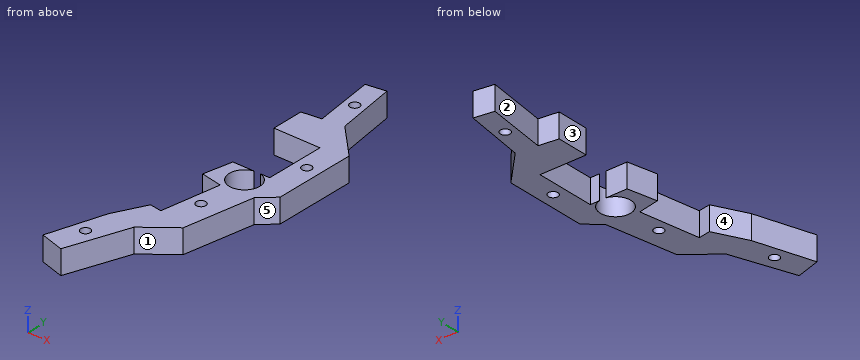
```python
from build123d import *

# Parameters (mm, degrees)
SKETCH1_R           = 1
BOSS_EXTRUDE1_DEPTH = 5
SKETCH2_R           = 3.2
CUT_EXTRUDE1_DEPTH  = 6


with BuildPart() as part:
    # Sketch1 → Boss-Extrude1 (new body)
    with BuildSketch(Plane.XY):
        Polygon((-30.344978495, 29.354997846), (-26.26481101, 29.998979434), (-24.229853855, 17.105806435), (-17.589395727, 10.355662433), (-17.589395727, -6.795999984), (-20.648203061, -9.632059779), (-23.169168461, -24.271324462), (-29.322804804, -29.218365444), (-33.858296815, -42.061599658), (-38.875160748, -40.557320866), (-35.210826338, -28.612806279), (-31.890475236, -22.08234188), (-29.422452502, -22.48091908), (-27.416937939, -10.06260833), (-31.846007079, -9.19781647), (-30.596587071, -3.168743327), (-22.846023992, -3.168743327), (-22.846023992, 9.3), (-32.534265366, 9.3), (-32.534265366, 15.998319193), (-28.533481358, 16.537502585), align=None)
        with Locations((-27.335083026, 23.255353238)):
            Circle(SKETCH1_R, mode=Mode.SUBTRACT)
        with Locations((-20.35, 3.1)):
            Circle(SKETCH1_R, mode=Mode.SUBTRACT)
        with Locations((-25.941584057, -16.567336204)):
            Circle(SKETCH1_R, mode=Mode.SUBTRACT)
        with Locations((-34.540975654, -35.117818403)):
            Circle(SKETCH1_R, mode=Mode.SUBTRACT)
    extrude(amount=BOSS_EXTRUDE1_DEPTH)

    # Sketch2 → Cut-Extrude1 (cut, through all)
    with BuildSketch(Plane(origin=(0, 0, 0), x_dir=(-1, 0, 0), z_dir=(0, 0, -1))):
        with Locations((25.5, -6.29339012)):
            Circle(SKETCH2_R)
    extrude(amount=-CUT_EXTRUDE1_DEPTH, mode=Mode.SUBTRACT)


solid = part.part
```
The model under review builds one solid part; all positions refer to its coordinate system, in mm. Face numbers are marked on the shaded views. A direction names the side the tool comes from. Give positions to 0.01 mm unless a question says otherwise; leave off trailing zeros. Write each loop counter-clockwise with the first axis right and the second up, starting at its lowest first coordinate (ties: lowest second). Pieces come first, ordered by that corner, then holes. Notation, with made-up numbers: M 87,38.25 L 136,38.25 A19 cw 136,59.25 Z; hole C 33.5,32 d9. An arc over 180 degrees is marked long. Write each question's results on one line, items separated by ' | '. Start each with the question number.
1. Mouldability with a two-part tool opening along Y and no side actions: class the marked faces 1, 2 and 3 as released by +Y, released by -Y, zero draft, split by the parting line, or undercut.
2. For probe 1 along X at (y, z) = (0, 2.5); probe 2 along Y at (x, z) = (-20.35, 1.55); probe 3 along Y at (x, z) = (-24, 2.65), list the stretches that pass through material, from the lowest coordinate up. Write a range as [from, to].
3. We need section B-B (z = 1.5). Count the separate pieces of the cut face and the enclosed holes in it, and give its area (3 significant figures).
4. Insertion check: pin 1 Ø2 at (y, z) = (-10, 0.5) entering from -X; pin 2 Ø1.5 at (x, z) = (-21, 1.5) entering from +Y (3 decimals); pin 3 Ø2.5 at (y, z) = (2.5, 2.5) entering from -X. Each pin has a flat end and moves straight along its axis. Give the tip position at first contact, or say it passes through.
5. For the marked faces 4 and 5, list the 3-axis set-ups (+Z, -Z, +X, -X, +Y, -Y) from which the entire face can be reached by the end or side of a thin tool; tool diameter is ignored.
6. We need section A-A (y = 3.1). Write out the cut boundary in (x, z), and give its area (3 significant figures).
7. We need section D-D (y = 20.5). Write out the cut boundary in (x, z).
8. We need section C-C (x = -37). Write out the cut boundary in (y, z), and give its area (3 significant figures).
Results found:
1) face 1: released by -Y | face 2: undercut | face 3: zero draft
2) probe 1: x = [-22.85, -17.59] | probe 2: y = [-9.36, 2.1], [4.1, 13.16] | probe 3: y = [-24.94, -9.12], [-3.47, -3.17], [9.3, 16.87]
3) separate pieces: 1 | enclosed holes: 4 | area: 462 mm^2
4) pin 1: stops at x = -31.85 | pin 2: stops at y = 14.585 | pin 3: stops at x = -22.85
5) face 4: +Z, -Z, -X | face 5: +Z, -Z, +X, -Y
6) outline: M -22.85,0 L -21.35,0 L -21.35,5 L -22.85,5 Z; M -19.35,0 L -17.59,0 L -17.59,5 L -19.35,5 Z | area: 16.3 mm^2
7) outline: M -29.09,0 L -24.77,0 L -24.77,5 L -29.09,5 Z
8) outline: M -41.12,0 L -34.44,0 L -34.44,5 L -41.12,5 Z | area: 33.4 mm^2
